from build123d import *

# Parameters (mm, degrees)
F0_W     = 236.205176
F0_H     = 266.267627
F0_W_2   = 180.947438
F1_DEPTH = 25.4
F2_W     = 317.041844
F2_H     = 415.295705
F3_DEPTH = 35.56


with BuildPart() as f1:
    # F0 (on Right) → F1 (new body)
    with BuildSketch(Plane.YZ):
        with Locations((-118.102588, 55.634335)):
            Rectangle(F0_W, F0_H)
        with Locations((90.473719, 55.634335)):
            Rectangle(F0_W_2, F0_H)
    extrude(amount=F1_DEPTH)

    # F2 (on Top) → F3 (join)
    with BuildSketch(Plane.XY):
        with Locations((-158.520922, -28.892569)):
            Rectangle(F2_W, F2_H)
    extrude(amount=F3_DEPTH)


solid = f1.part
The listing builds one solid part. Answer for the finished solid, in the listing's coordinates (mm). A direction names the side the tool comes from. Give positions to 0.01 mm unless a question says otherwise; leave off trailing zeros. Loops run counter-clockwise (first coordinate to the right, second up) from the corner with the lowest first, then second, coordinate; pieces in that order, holes last.
Item 1: Each of these flat-tipped pins is pushed along its axis until it touches: pin 1 Ø10.5 at (x, z) = (-155, 13) entering from +Y; pin 2 Ø7.5 at (x, z) = (9.5, 66.5) entering from -Y; pin 3 Ø12 at (x, y) = (-47, -7.5) entering from -Z. Where does it stop, or does it pass through?
Derived:
pin 1: stops at y = 178.76
pin 2: stops at y = -236.21
pin 3: stops at z = 0
Item 2: A tool of negligible diameter and unlimited length cuts with its end or side. For faces 1 (the flat face through (25.4, -31, 57)), 2 (the flat face through (-161, -26, 0)), 3 (the flat face through (-161, 178.755, 18)), 4 (the flat face through (-161, -26, 35.56)), from which of +Z, -Z, +X, -X, +Y, -Y can it reach the whole face along a straight path? Write none if from no direction.
Derived:
face 1: +Z, -Z, +X, +Y, -Y
face 2: -Z, -X, +Y, -Y
face 3: +Z, -Z, -X, +Y
face 4: +Z, -X, +Y, -Y
Item 3: A cutting plane is placed at A-A (y = 17). Give the vertices of the cut face in (x, z).
Derived:
outline: (-317.04, 0) - (0, 0) - (0, -77.5) - (25.4, -77.5) - (25.4, 188.77) - (0, 188.77) - (0, 35.56) - (-317.04, 35.56) - close
Item 4: Find the intervals of material crossed by line 1 along Z through (x, y) = (-246.5, 119); line 2 along Y through (x, z) = (-41.5, 17); line 3 along X through (y, z) = (-78, 42.5), in increasing order.
Derived:
line 1: z = 0 to 35.56
line 2: y = -236.54 to 178.76
line 3: x = 0 to 25.4
Item 5: A cutting plane is placed at B-B (z = -11). Give the vertices of the cut face in (x, y), then the cut area to 3 significant figures.
Derived:
outline: (0, -236.21) - (25.4, -236.21) - (25.4, 180.95) - (0, 180.95) - close
area: 10,600 mm2
Item 6: A cutting plane is placed at C-C (x = -136.5). Give the vertices of the cut face in (y, z), then the cut area to 3 significant figures.
Derived:
outline: (-236.54, 0) - (178.76, 0) - (178.76, 35.56) - (-236.54, 35.56) - close
area: 14,800 mm2
